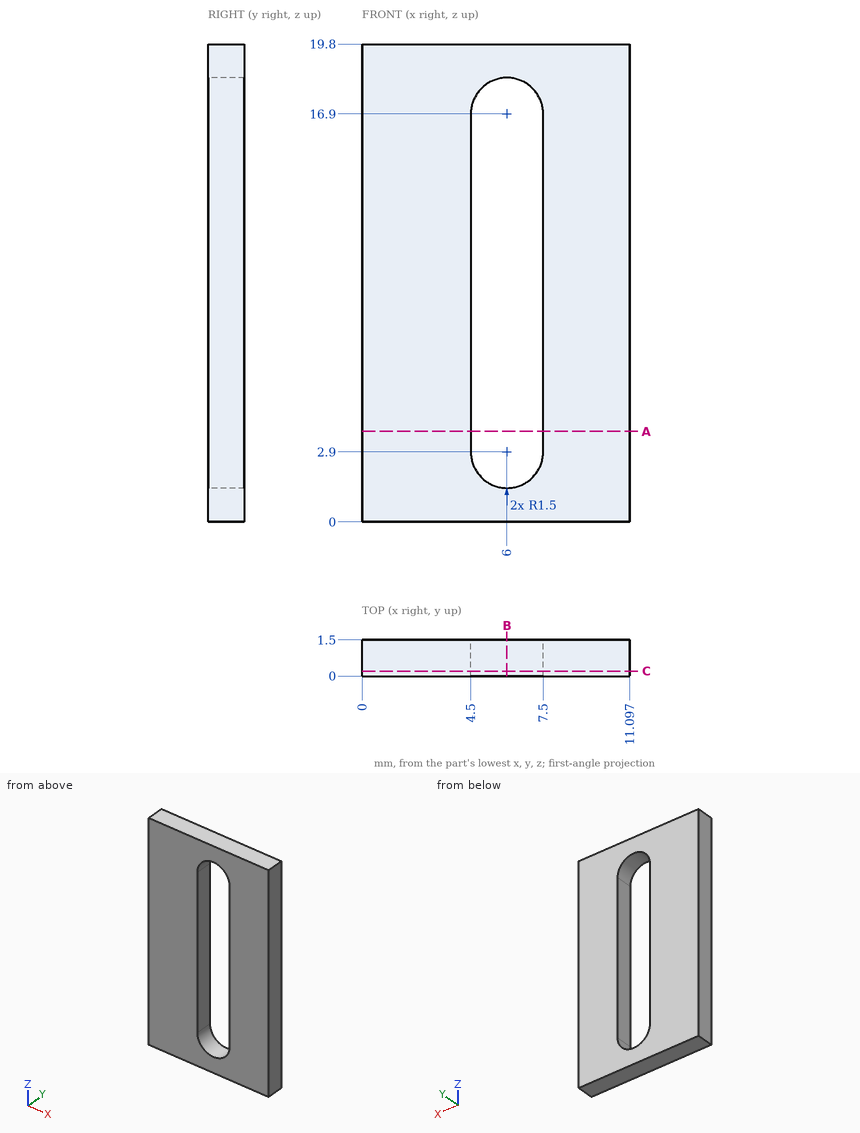
Check sheet for the drawn part. Datum: minimum x, y, z corner. Units: mm. Round coordinates to 2 decimals unless told otherwise and drop trailing zeros. Order: outer loops, then holes, each group sorted by start corner. A loop starts at its lowest first (then second) coordinate and runs counter-clockwise, first axis right, second up. Notation, with made-up numbers: M 85.25,-33.5 L 138.25,-33.5 A25 cw 138.25,-15.5 Z; hole C 46,56.5 d2. An arc over 180 degrees is marked long. Write each question's results on one line, items separated by ' | '. Start each with the question number.
1. Cross-section at C-C on y = 0.2. Record the boundary of the cut face in (x, z), plus the area to 3 significant figures.
2. Material ranges on L1, parallel to X at y = 1.2, z = 12; L2, parallel to Z at x = 6, y = 1.2; L3, parallel to X at y = 1.1, z = 17.5 (1 decimal), recorded low to high. Write a range as from..to.
3. Cross-section at A-A on z = 3.75. Record the boundary of the cut face in (x, y).
4. Cross-section at B-B on x = 6. Record the boundary of the cut face in (y, z).
Resolved:
1) outline: M 0,0 L 11.1,0 L 11.1,19.8 L 0,19.8 Z; hole M 4.5,2.9 A1.5 ccw 7.5,2.9 L 7.5,16.9 A1.5 ccw 4.5,16.9 Z | area: 171 mm2
2) L1: 0..4.5, 7.5..11.1 | L2: 0..1.4, 18.4..19.8 | L3: 0..4.6, 7.4..11.1
3) outline: M 0,0 L 4.5,0 L 4.5,1.5 L 0,1.5 Z; M 7.5,0 L 11.1,0 L 11.1,1.5 L 7.5,1.5 Z
4) outline: M 0,0 L 1.5,0 L 1.5,1.4 L 0,1.4 Z; M 0,18.4 L 1.5,18.4 L 1.5,19.8 L 0,19.8 Z
